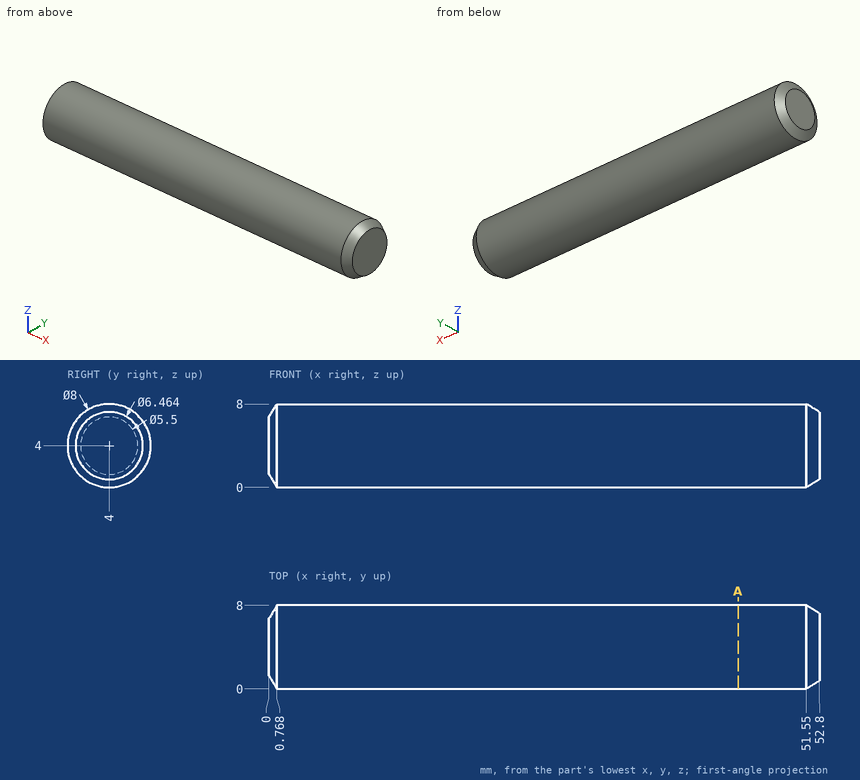
Job drawing, mm, ordinate dimensions from the low corner. One solid piece. Round coordinates to 2 decimals unless told otherwise and drop trailing zeros. Order: outer loops, then holes, each group sorted by start corner. A loop starts at its lowest first (then second) coordinate and runs counter-clockwise, first axis right, second up. Notation, with made-up numbers: (-16, 26.25) -> (11, 26.25) arc R10 cw to (11, 35.25) -> close; hole circle Ø9 at (-36.5, 51.5). An arc over 180 degrees is marked (long way). Write item = value, one per line.
(1) Cut at A-A (x = 45). Write the cut outline in (y, z).
Answers follow:
outline = circle Ø8 at (4, 4)
(2) Drill centre lines: L1, parallel to Y at x = 37, z = 1.25 (1 decimal); L2, parallel to Y at x = 7.5, z = 2.5; L3, parallel to X at y = 6.5, z = 5.25. Where is each one in solid material? Low to high.
Answers follow:
L1 = 1.1 to 6.9
L2 = 0.29 to 7.71
L3 = 0.03 to 52.8
(3) Flat gauge pins, fed straight in: P1, Ø1, axis at x = 33, z = 6, coming from the +Y side; P2, Ø3, axis at x = 10, z = 2, coming from the +Y side. Where does each tip first touch, or does it go through?
Answers follow:
P1 = 7.71
P2 = 7.97
